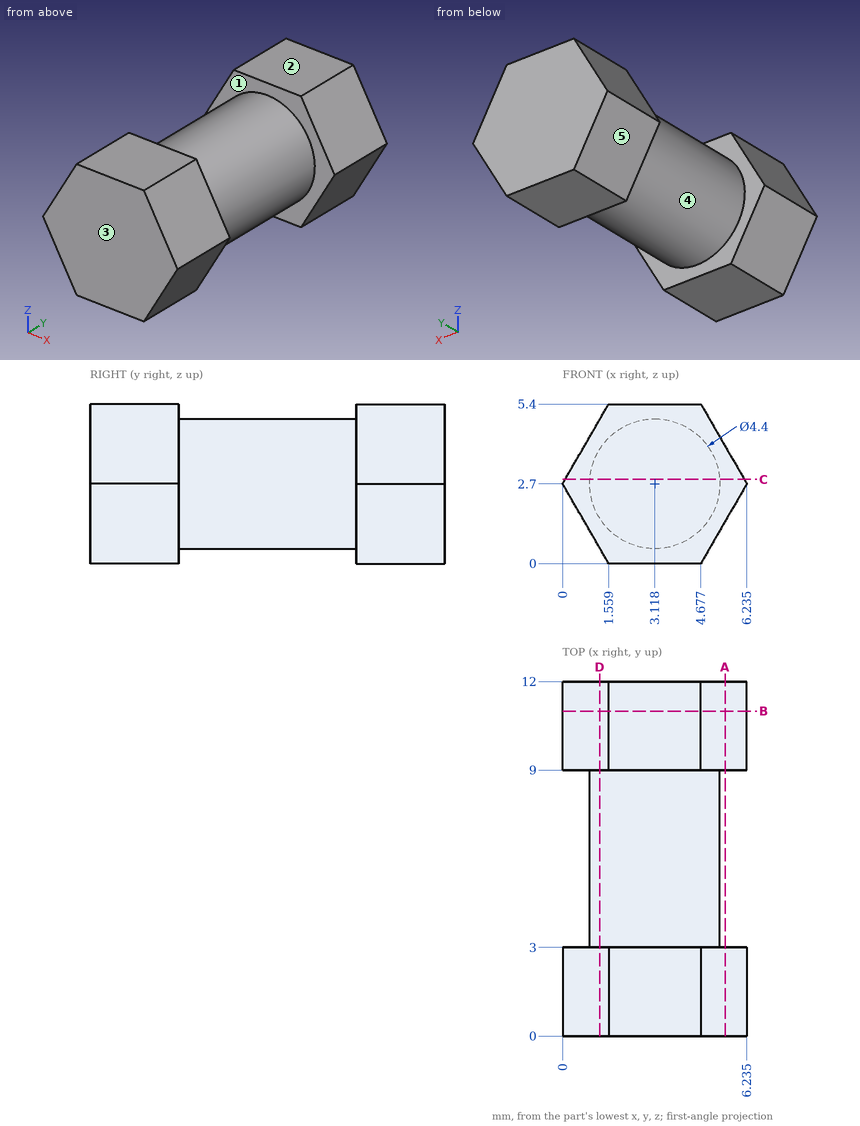
Source: three-view drawing plus pictorial views. Frame: mm from the lowest corner of the part. A direction names the side the tool comes from. Round coordinates to 2 decimals unless told otherwise and drop trailing zeros. Write each loop counter-clockwise with the first axis right and the second up, starting at its lowest first coordinate (ties: lowest second). Pieces come first, ordered by that corner, then holes. Notation, with made-up numbers: M 1.25,47.25 L 50.25,47.25 A15 ccw 50.25,73.25 Z; hole C 47.5,-17.5 d8. An arc over 180 degrees is marked long. Use CSV: the item, a comma, the result in double quotes. Start each with the question number.
Q1. First-contact query: P1, Ø1.5, axis at x = 4.5, y = 7, coming from the +Z side. Flat tip, straight axial feed; report the tip coordinate or a pass-through.
Q2. Cut plane D-D on x = 1.25. Output: boundary loops of the cut face in (y, z) (1 decimal).
Q3. Cut plane C-C on z = 2.85. Output: boundary loops of the cut face in (x, y), plus the area to 3 significant figures.
Q4. Cut plane A-A on x = 5.5. Output: boundary loops of the cut face in (y, z), plus the area to 3 significant figures.
Q5. Pull-direction query (Y, two-part tool) for the marked faces 3, 4 and 5; classes: +Y half, -Y half, draft (parallel to the pull), parting line (faces both ways), or undercut.
Q6. Cut plane B-B on y = 11. Output: boundary loops of the cut face in (x, z) (1 decimal).
Q7. Line query: line 1 (Y direction, x = 5.5, z = 3.3); line 2 (X direction, y = 4, z = 4.1) (1 decimal); line 3 (Z direction, x = 1.5, y = 2.75) (1 decimal). Output: solid intervals per line, ascending. Write a range as from..to.
Q8. Access query for the marked faces 1 and 2. Directions: +Z, -Z, +X, -X, +Y, -Y. A direction counts if a zero-diameter tool reaches every point of the face in a straight line with its end or side. Return the directions, or none.
Results found:
1,P1,"z = 4.81"
2,outline,"M 0,0.5 L 3,0.5 L 3,1.5 L 9,1.5 L 9,0.5 L 12,0.5 L 12,4.9 L 9,4.9 L 9,3.9 L 3,3.9 L 3,4.9 L 0,4.9 Z"
3,outline,"M 0.09,0 L 6.15,0 L 6.15,3 L 5.31,3 L 5.31,9 L 6.15,9 L 6.15,12 L 0.09,12 L 0.09,9 L 0.92,9 L 0.92,3 L 0.09,3 Z"
3,area,"62.7 mm^2"
4,outline,"M 0,1.43 L 3,1.43 L 3,3.97 L 0,3.97 Z; M 9,1.43 L 12,1.43 L 12,3.97 L 9,3.97 Z"
4,area,"15.3 mm^2"
5,face 3,"-Y half"
5,face 4,"undercut"
5,face 5,"draft"
6,outline,"M 0,2.7 L 1.6,0 L 4.7,0 L 6.2,2.7 L 4.7,5.4 L 1.6,5.4 Z"
7,line 1,"0..3, 9..12"
7,line 2,"1.4..4.8"
7,line 3,"0.1..5.3"
8,face 1,"none"
8,face 2,"+Z, +X, -X, +Y, -Y"
